The drawing under review shows one solid part. Ordinate dimensions are in mm from its lowest x, y, z. A direction names the side the tool comes from. Coordinates: 2 decimals unless noted, no trailing zeros. Loops run counter-clockwise (first coordinate to the right, second up) from the corner with the lowest first, then second, coordinate; pieces in that order, holes last. Notation, with made-up numbers: (44.25, 80.25) -> (99.25, 80.25) arc R31 ccw to (99.25, 104.25) -> close; hole circle Ø3 at (28, -10). An arc over 180 degrees is marked (long way). Use a Markdown table: item, result.
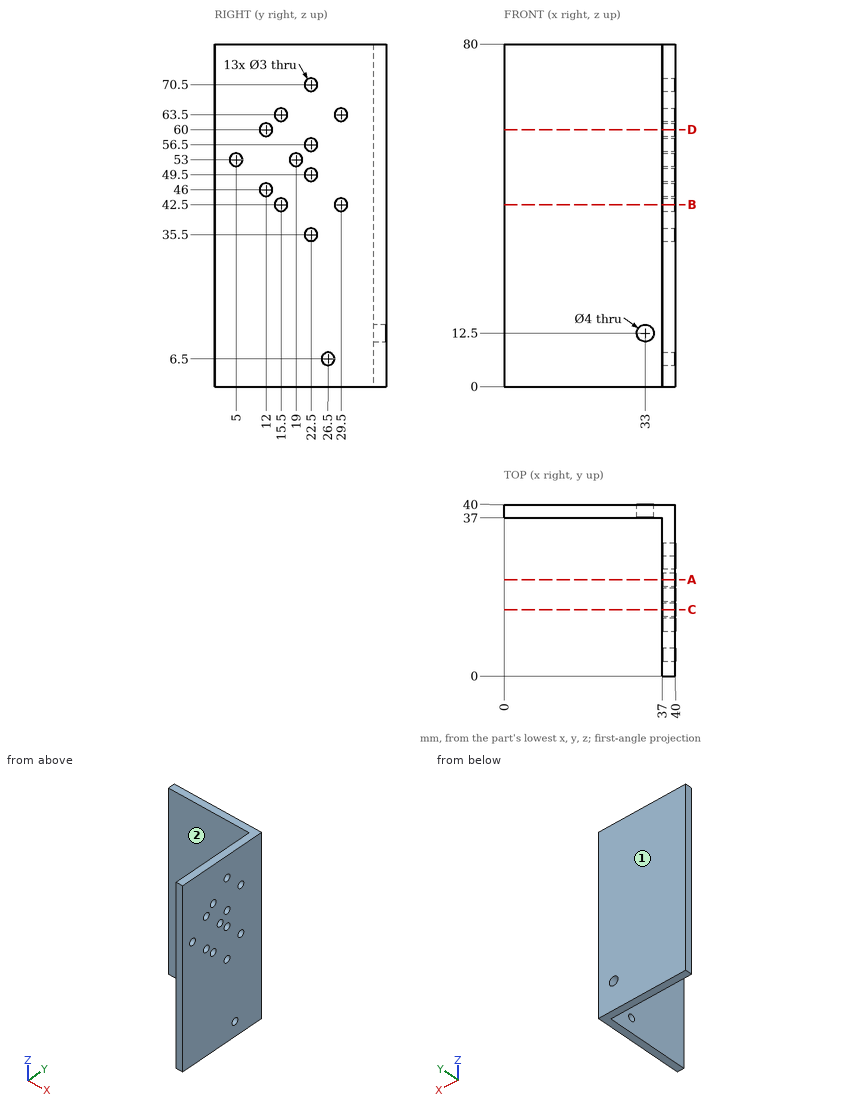
(1) Take a section at A-A on y = 22.5. Write out the cut boundary in (x, z).
Found:
| item | result |
|---|---|
| outline | (37, 0) -> (40, 0) -> (40, 34) -> (37, 34) -> close; (37, 37) -> (40, 37) -> (40, 48) -> (37, 48) -> close; (37, 51) -> (40, 51) -> (40, 55) -> (37, 55) -> close; (37, 58) -> (40, 58) -> (40, 69) -> (37, 69) -> close; (37, 72) -> (40, 72) -> (40, 80) -> (37, 80) -> close |
(2) For the marked faces 1 and 2, list the 3-axis set-ups (+Z, -Z, +X, -X, +Y, -Y) from which the entire face can be reached by the end or side of a thin tool; tool diameter is ignored.
Found:
| item | result |
|---|---|
| face 1 | +Z, -Z, +X, -X, +Y |
| face 2 | +Z, -Z, -X, -Y |
(3) Take a section at C-C on y = 15.5. Write out the cut boundary in (x, z), plus the area to 3 significant figures.
Found:
| item | result |
|---|---|
| outline | (37, 0) -> (40, 0) -> (40, 41) -> (37, 41) -> close; (37, 44) -> (40, 44) -> (40, 62) -> (37, 62) -> close; (37, 65) -> (40, 65) -> (40, 80) -> (37, 80) -> close |
| area | 222 mm^2 |
(4) For pin 1 Ø11 at (x, z) = (9.5, 51.5) entering from -Y; pin 2 Ø5 at (y, z) = (22.5, 49.5) entering from -X; pin 3 Ø3 at (x, z) = (33, 12.5) entering from +Y, all flat-tipped, find the tip position at first contact; note any pin that passes through.
Found:
| item | result |
|---|---|
| pin 1 | stops at y = 37 |
| pin 2 | stops at x = 37 |
| pin 3 | passes through |
(5) Take a section at D-D on z = 60. Write out the cut boundary in (x, y), plus the area to 3 significant figures.
Found:
| item | result |
|---|---|
| outline | (0, 37) -> (37, 37) -> (37, 13.5) -> (40, 13.5) -> (40, 40) -> (0, 40) -> close; (37, 0) -> (40, 0) -> (40, 10.5) -> (37, 10.5) -> close |
| area | 222 mm^2 |
(6) Take a section at B-B on z = 42.5. Write out the cut boundary in (x, y), plus the area to 3 significant figures.
Found:
| item | result |
|---|---|
| outline | (0, 37) -> (37, 37) -> (37, 31) -> (40, 31) -> (40, 40) -> (0, 40) -> close; (37, 0) -> (40, 0) -> (40, 14) -> (37, 14) -> close; (37, 17) -> (40, 17) -> (40, 28) -> (37, 28) -> close |
| area | 213 mm^2 |
(7) For line 1 along Z through (x, y) = (38.8, 22.5); line 2 along Z through (x, y) = (39.4, 5); line 3 along X through (y, z) = (39.25, 12.5), list the stretches that pass through material, from the lowest coordinate up.
Found:
| item | result |
|---|---|
| line 1 | z = 0 to 34, 37 to 48, 51 to 55, 58 to 69, 72 to 80 |
| line 2 | z = 0 to 51.5, 54.5 to 80 |
| line 3 | x = 0 to 31, 35 to 40 |
